Geometry: final body of the model. Coordinates: model frame, mm. Face numbers are marked on the shaded views. A direction names the side the tool comes from. Give positions to 0.01 mm unless a question says otherwise; leave off trailing zeros. Loops run counter-clockwise (first coordinate to the right, second up) from the corner with the lowest first, then second, coordinate; pieces in that order, holes last. Notation, with made-up numbers: (64, -7.75) - (75, -7.75) arc R22 cw to (75, 31.25) - close; hole circle Ø6 at (48, 54.25). An arc over 180 degrees is marked (long way). Use one line per item in the form item = value.
```python
from build123d import *

# Parameters (mm, degrees)
SKETCH1_W           = 34.0614
SKETCH1_H           = 32.512
BOSS_EXTRUDE1_DEPTH = 8.9916
SKETCH2_W           = 34.0614
SKETCH2_H           = 12.065
BOSS_EXTRUDE2_DEPTH = 13.97
SKETCH3_W           = 17.0307
SKETCH3_H           = 12.065
REVOLVE1_ANGLE      = 180
SKETCH4_R           = 2.0955
CUT_EXTRUDE1_DEPTH  = 7.62
CUT_EXTRUDE2_REACH  = 10.992
SKETCH5_R           = 2.7686
SKETCH5_R_2         = 2.6416


with BuildPart() as part:
    # Sketch1 → Boss-Extrude1 (new body)
    with BuildSketch(Plane(origin=(0, 0, 0), x_dir=(0, 0, -1), z_dir=(1, 0, 0))):
        Rectangle(SKETCH1_W, SKETCH1_H)
    extrude(amount=BOSS_EXTRUDE1_DEPTH)

    # Sketch2 → Boss-Extrude2 (add)
    with BuildSketch(Plane(origin=(8.9916, 0, 0), x_dir=(0, 0, -1), z_dir=(1, 0, 0))):
        with Locations((0, 10.2235)):
            Rectangle(SKETCH2_W, SKETCH2_H)
    extrude(amount=BOSS_EXTRUDE2_DEPTH)

    # Sketch3 → Revolve1 (revolve)
    with BuildSketch(Plane(origin=(22.9616, 0, 0), x_dir=(0, 0, -1), z_dir=(1, 0, 0))):
        with Locations((8.51535, 10.2235)):
            Rectangle(SKETCH3_W, SKETCH3_H)
    revolve(axis=Axis((22.9616, 16.256, 0), (0, -1, 0)), revolution_arc=REVOLVE1_ANGLE)

    # Sketch4 → Cut-Extrude1 (cut)
    with BuildSketch(Plane(origin=(0, 16.256, 0), x_dir=(1, 0, 0), z_dir=(0, 1, 0))):
        with Locations((22.9616, 0)):
            Circle(SKETCH4_R)
    extrude(amount=-CUT_EXTRUDE1_DEPTH, mode=Mode.SUBTRACT)

    # Sketch5 → Cut-Extrude2 (cut, up to next)
    with BuildSketch(Plane(origin=(8.9916, 0, 0), x_dir=(0, 0, -1), z_dir=(1, 0, 0)), mode=Mode.PRIVATE) as cut_extrude2_sk1:
        with Locations((-10.0076, -6.0325)):
            Circle(SKETCH5_R)
    cut_extrude2_tool1 = extrude(cut_extrude2_sk1.sketch, amount=-CUT_EXTRUDE2_REACH, mode=Mode.PRIVATE) & part.part
    add(cut_extrude2_tool1.solids().sort_by_distance((8.9916, -6.0325, 10.0076))[0], mode=Mode.SUBTRACT)
    # Sketch5 → Cut-Extrude2 (cut, up to next)
    with BuildSketch(Plane(origin=(8.9916, 0, 0), x_dir=(0, 0, -1), z_dir=(1, 0, 0)), mode=Mode.PRIVATE) as cut_extrude2_sk2:
        with Locations((10.0076, -6.0325)):
            Circle(SKETCH5_R_2)
    cut_extrude2_tool2 = extrude(cut_extrude2_sk2.sketch, amount=-CUT_EXTRUDE2_REACH, mode=Mode.PRIVATE) & part.part
    add(cut_extrude2_tool2.solids().sort_by_distance((8.9916, -6.0325, -10.0076))[0], mode=Mode.SUBTRACT)


solid = part.part
```
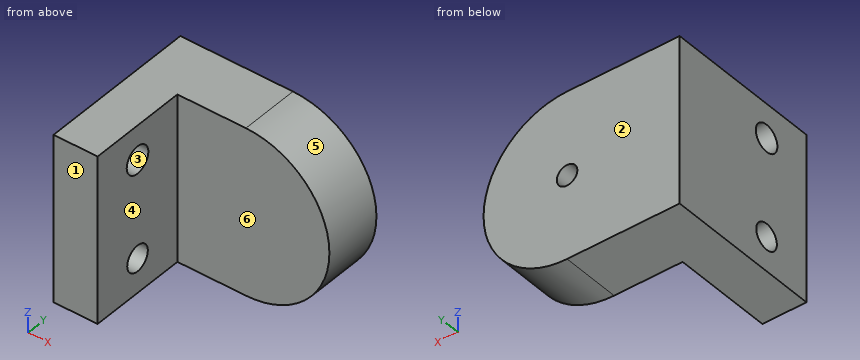
(1) Pin query (flat end, axial travel): P1, Ø6, axis at x = 35.5, y = 0, coming from the -Z side; P2, Ø9.5, axis at x = 28.5, z = -8, coming from the -Y side; P3, Ø10, axis at y = 12.5, z = 6, coming from the -X side; P4, Ø10, axis at y = 12.5, z = 5.5, coming from the +X side. Return the tip coordinate at first contact, or that it passes through.
Solution:
P1 = through
P2 = 4.19
P3 = 0
P4 = 39.98
(2) Cut plane D-D (z = -12). Return the cut outline in (x, y).
Solution:
outline = (0, -16.26) - (8.99, -16.26) - (8.99, -7.77) - (0, -7.77) - close; (0, -4.3) - (8.99, -4.3) - (8.99, 4.19) - (35.05, 4.19) - (35.05, 16.26) - (0, 16.26) - close
(3) Pull-direction query (Y, two-part tool) for the marked faces 1, 2, 3 and 4; classes: released by +Y, released by -Y, zero draft, split by the parting line, or undercut.
Solution:
face_1 = released by -Y
face_2 = released by +Y
face_3 = undercut
face_4 = zero draft
(4) Access query for the marked faces 5 and 6. Directions: +Z, -Z, +X, -X, +Y, -Y. A direction counts if a zero-diameter tool reaches every point of the face in a straight line with its end or side. Return the directions, or none.
Solution:
face_5 = +X, +Y, -Y
face_6 = +Z, -Z, +X, -Y
(5) Material intervals for L1, parallel to X at y = 13, z = 0; L2, parallel to Z at x = 7, y = -4.5; L3, parallel to X at y = 4, z = 14.5, sorted ascending. Write a range as from..to.
Solution:
L1 = 0..20.87, 25.06..39.99
L2 = -17.03..-12.16, -7.86..7.7, 12.31..17.03
L3 = 0..8.99
(6) Cut plane C-C (x = 6.5). Return the cut outline in (y, z).
Solution:
outline = (-16.26, -17.03) - (16.26, -17.03) - (16.26, 17.03) - (-16.26, 17.03) - close; hole circle Ø5.54 at (-6.03, 10.01); hole circle Ø5.28 at (-6.03, -10.01)
(7) Cut plane A-A (y = -7). Return the cut outline in (x, z).
Solution:
outline = (0, -17.03) - (8.99, -17.03) - (8.99, -12.47) - (0, -12.47) - close; (0, -7.55) - (8.99, -7.55) - (8.99, 7.41) - (0, 7.41) - close; (0, 12.6) - (8.99, 12.6) - (8.99, 17.03) - (0, 17.03) - close
(8) Cut plane B-B (z = 0). Return the cut outline in (x, y), plus the area to 3 significant figures.
Solution:
outline = (0, -16.26) - (8.99, -16.26) - (8.99, 4.19) - (39.99, 4.19) - (39.99, 16.26) - (25.06, 16.26) - (25.06, 8.64) - (20.87, 8.64) - (20.87, 16.26) - (0, 16.26) - close
area = 634 mm2
